```python
from build123d import *

# Parameters (mm, degrees)
F1_DEPTH = 10
F2_DEPTH = 7.95
F3_DEPTH = 2.5
F4_R     = 1.0622539674


with BuildPart() as f1:
    # F0 (on Front) → F1 (new body)
    with BuildSketch(Plane.XZ):
        with BuildLine():
            ThreePointArc((10.6592367905, -2.7167390458), (10.9144767327, -1.3690133864), (11, 0))
            ThreePointArc((11, 0), (10.9127641391, 1.3825985843), (10.65244021, 2.7432676816))
            Line((10.65244021, 2.7432676816), (9.2721758837, 2.9730035594))
            Line((9.2721758837, 2.9730035594), (10.2124558135, 4.0872663551))
            ThreePointArc((10.2124558135, 4.0872663551), (8.8785549643, 6.4939403867), (6.9890934799, 8.4942670272))
            Line((6.9890934799, 8.4942670272), (5.7386160604, 7.8664020679))
            Line((5.7386160604, 7.8664020679), (5.8415511192, 9.3207446335))
            ThreePointArc((5.8415511192, 9.3207446335), (3.3455445115, 10.4788993659), (0.6401960862, 10.9813546055))
            Line((0.6401960862, 10.9813546055), (0, 9.7371451557))
            Line((0, 9.7371451557), (-0.7739624833, 10.9727381302))
            ThreePointArc((-0.7739624833, 10.9727381302), (-3.3716222336, 10.4705378808), (-5.7742283081, 9.3626004638))
            Line((-5.7742283081, 9.3626004638), (-5.5849970186, 7.9762023598))
            Line((-5.5849970186, 7.9762023598), (-6.9276969841, 8.5444142278))
            ThreePointArc((-6.9276969841, 8.5444142278), (-8.8315250081, 6.5577561735), (-10.1827352173, 4.1607575626))
            Line((-10.1827352173, 4.1607575626), (-9.2127819423, 3.1522443856))
            Line((-9.2127819423, 3.1522443856), (-10.6323938835, 2.819964593))
            ThreePointArc((-10.6323938835, 2.819964593), (-10.9996071509, 0.0929651823), (-10.6785385121, -2.6398513682))
            Line((-10.6785385121, -2.6398513682), (-9.300566617, -2.8829596573))
            Line((-9.300566617, -2.8829596573), (-10.2516063733, -3.9880530046))
            ThreePointArc((-10.2516063733, -3.9880530046), (-8.941103633, -6.407547567), (-7.0711263799, -8.4261006236))
            Line((-7.0711263799, -8.4261006236), (-5.8146198884, -7.8103899606))
            Line((-5.8146198884, -7.8103899606), (-5.9316515908, -9.2636660888))
            ThreePointArc((-5.9316515908, -9.2636660888), (-3.4469919259, -10.445967962), (-0.7466425421, -10.9746309694))
            Line((-0.7466425421, -10.9746309694), (-0.0944125443, -9.7366874272))
            Line((-0.0944125443, -9.7366874272), (0.6675330963, -10.9797267528))
            ThreePointArc((0.6675330963, -10.9797267528), (3.3716222336, -10.4705378808), (5.8647377838, -9.3061727218))
            Line((5.8647377838, -9.3061727218), (5.662072705, -7.9216745998))
            Line((5.662072705, -7.9216745998), (7.0102190036, -8.4768407748))
            ThreePointArc((7.0102190036, -8.4768407748), (8.8946946533, -6.4718163621), (10.2225997539, -4.0618289319))
            Line((10.2225997539, -4.0618289319), (9.2429134084, -3.0627679486))
            Line((9.2429134084, -3.0627679486), (10.6592367905, -2.7167390458))
        make_face()
        with BuildLine():
            ThreePointArc((0.65, 3.7947331922), (2.9432125306, 2.4819347292), (3.85, 0))
            ThreePointArc((3.85, 0), (2.9432125306, -2.4819347292), (0.65, -3.7947331922))
            ThreePointArc((0.65, -3.7947331922), (-3.85, 0), (0.65, 3.7947331922))
        make_face(mode=Mode.SUBTRACT)
    extrude(amount=F1_DEPTH)

    # F0 (on Front) → F2 (join)
    with BuildSketch(Plane.XZ):
        with BuildLine():
            ThreePointArc((0.65, -3.7947331922), (2.9432125306, -2.4819347292), (3.85, 0))
            ThreePointArc((3.85, 0), (2.9432125306, 2.4819347292), (0.65, 3.7947331922))
            Line((0.65, 3.7947331922), (0.65, -3.7947331922))
        make_face()
    extrude(amount=F2_DEPTH)

    # F0 (on Front) → F3 (join)
    with BuildSketch(Plane.XZ):
        with BuildLine():
            ThreePointArc((10.6592367905, -2.7167390458), (10.9144767327, -1.3690133864), (11, 0))
            ThreePointArc((11, 0), (10.9127641391, 1.3825985843), (10.65244021, 2.7432676816))
            Line((10.65244021, 2.7432676816), (9.2721758837, 2.9730035594))
            Line((9.2721758837, 2.9730035594), (10.2124558135, 4.0872663551))
            ThreePointArc((10.2124558135, 4.0872663551), (8.8785549643, 6.4939403867), (6.9890934799, 8.4942670272))
            Line((6.9890934799, 8.4942670272), (5.7386160604, 7.8664020679))
            Line((5.7386160604, 7.8664020679), (5.8415511192, 9.3207446335))
            ThreePointArc((5.8415511192, 9.3207446335), (3.3455445115, 10.4788993659), (0.6401960862, 10.9813546055))
            Line((0.6401960862, 10.9813546055), (0, 9.7371451557))
            Line((0, 9.7371451557), (-0.7739624833, 10.9727381302))
            ThreePointArc((-0.7739624833, 10.9727381302), (-3.3716222336, 10.4705378808), (-5.7742283081, 9.3626004638))
            Line((-5.7742283081, 9.3626004638), (-5.5849970186, 7.9762023598))
            Line((-5.5849970186, 7.9762023598), (-6.9276969841, 8.5444142278))
            ThreePointArc((-6.9276969841, 8.5444142278), (-8.8315250081, 6.5577561735), (-10.1827352173, 4.1607575626))
            Line((-10.1827352173, 4.1607575626), (-9.2127819423, 3.1522443856))
            Line((-9.2127819423, 3.1522443856), (-10.6323938835, 2.819964593))
            ThreePointArc((-10.6323938835, 2.819964593), (-10.9996071509, 0.0929651823), (-10.6785385121, -2.6398513682))
            Line((-10.6785385121, -2.6398513682), (-9.300566617, -2.8829596573))
            Line((-9.300566617, -2.8829596573), (-10.2516063733, -3.9880530046))
            ThreePointArc((-10.2516063733, -3.9880530046), (-8.941103633, -6.407547567), (-7.0711263799, -8.4261006236))
            Line((-7.0711263799, -8.4261006236), (-5.8146198884, -7.8103899606))
            Line((-5.8146198884, -7.8103899606), (-5.9316515908, -9.2636660888))
            ThreePointArc((-5.9316515908, -9.2636660888), (-3.4469919259, -10.445967962), (-0.7466425421, -10.9746309694))
            Line((-0.7466425421, -10.9746309694), (-0.0944125443, -9.7366874272))
            Line((-0.0944125443, -9.7366874272), (0.6675330963, -10.9797267528))
            ThreePointArc((0.6675330963, -10.9797267528), (3.3716222336, -10.4705378808), (5.8647377838, -9.3061727218))
            Line((5.8647377838, -9.3061727218), (5.662072705, -7.9216745998))
            Line((5.662072705, -7.9216745998), (7.0102190036, -8.4768407748))
            ThreePointArc((7.0102190036, -8.4768407748), (8.8946946533, -6.4718163621), (10.2225997539, -4.0618289319))
            Line((10.2225997539, -4.0618289319), (9.2429134084, -3.0627679486))
            Line((9.2429134084, -3.0627679486), (10.6592367905, -2.7167390458))
        make_face()
        with BuildLine():
            ThreePointArc((0.65, 3.7947331922), (2.9432125306, 2.4819347292), (3.85, 0))
            ThreePointArc((3.85, 0), (2.9432125306, -2.4819347292), (0.65, -3.7947331922))
            ThreePointArc((0.65, -3.7947331922), (-3.85, 0), (0.65, 3.7947331922))
        make_face(mode=Mode.SUBTRACT)
        with BuildLine():
            Line((0.65, -3.7947331922), (0.65, 3.7947331922))
            ThreePointArc((0.65, 3.7947331922), (-3.85, 0), (0.65, -3.7947331922))
        make_face()
        with BuildLine():
            ThreePointArc((0.65, -3.7947331922), (2.9432125306, -2.4819347292), (3.85, 0))
            ThreePointArc((3.85, 0), (2.9432125306, 2.4819347292), (0.65, 3.7947331922))
            Line((0.65, 3.7947331922), (0.65, -3.7947331922))
        make_face()
    extrude(amount=-F3_DEPTH)

    # F4
    f4_edges = [f1.edges().sort_by_distance(p)[0] for p in [
        (-3.446992, 2.5, -10.445968),
        (3.371622, 2.5, -10.470538),
        (8.878555, 2.5, 6.49394),
        (3.345545, 2.5, 10.478899),
        (-3.371622, 2.5, 10.470538),
        (-8.831525, 2.5, 6.557756),
        (-10.999607, 2.5, 0.092965),
        (-8.941104, 2.5, -6.407548),
        (8.894695, 2.5, -6.471816),
        (10.999991, 2.5, 0.013693),
    ]]
    fillet(f4_edges, radius=F4_R)


solid = f1.part
```
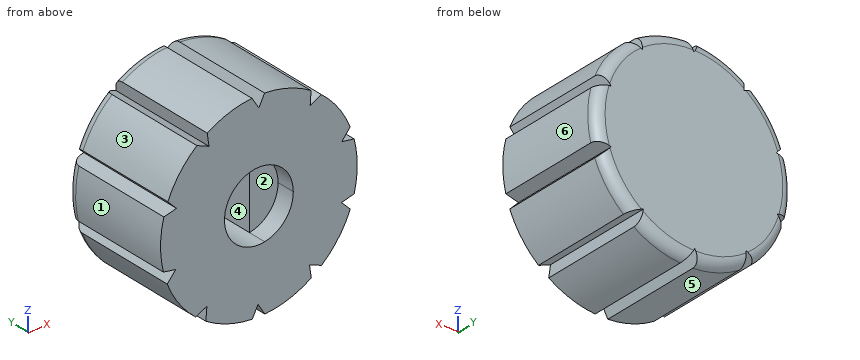
Check sheet for the modelled part. Datum: model origin and axes. Units: mm. Face numbers are marked on the shaded views. A direction names the side the tool comes from. Give positions to 0.01 mm unless a question says otherwise; leave off trailing zeros. Answer as a JSON object with one key per item and string values. Group by question number.
1) Thickness scan on probe 1 along X at (y, z) = (-2.5, 0); probe 2 along Z at (x, y) = (0.25, -1). Record the ranges inside material, lowest first. Write a range as from..to.
2) Release check for a two-part mould opening along Z. For the marked faces 3, 4, 5 and 6 record: pulls with the +Z half, pulls with the -Z half, needs draft (parallel to the pull), parting line crosses it, or undercut.
3) Access from +Z, -Z, +X, -X, +Y, -Y to the whole of each face (thin tool, end or side, straight path). Record for the marked faces 1 and 2.
4) Depth check by flat-ended pin: P1, Ø3, axis at y = -6, z = -4.5, coming from the +X side; P2, Ø1, axis at x = 3, z = -0.5, coming from the -Y side; P3, Ø5, axis at x = 6, y = -0.5, coming from the -Z side. Enter the tip coordinate at first touch or a pass-through.
Geometry results:
{
 "1": {"probe 1": "x = -11..-3.85, 0.65..11", "probe 2": "z = -10.3..-3.84, 3.84..10.22"},
 "2": {"face 3": "pulls with the +Z half", "face 4": "undercut", "face 5": "pulls with the -Z half", "face 6": "parting line crosses it"},
 "3": {"face 1": "-X, +Y, -Y", "face 2": "-Y"},
 "4": {"P1": "stops at x = 10.22", "P2": "stops at y = -7.95", "P3": "stops at z = -10.43"}
}
